```python
from build123d import *

# Parameters (mm, degrees)
CROQUIS1_R              = 1.75
SALIENTE_EXTRUIR1_DEPTH = 3
SALIENTE_EXTRUIR3_DEPTH = 10
CROQUIS4_W              = 70.682064062
CROQUIS4_H              = 54
CORTAR_EXTRUIR1_DEPTH   = 1.5


with BuildPart() as part:
    # Croquis1 → Saliente-Extruir1 (new body)
    with BuildSketch(Plane(origin=(0, 0, 0), x_dir=(1, 0, 0), z_dir=(0, 1, 0))):
        with BuildLine():
            Line((0, 35), (-75, 35))
            Line((-75, 35), (-75, -35))
            Line((-75, -35), (0, -35))
            ThreePointArc((0, -35), (35, 0), (0, 35))
        make_face()
        with Locations(Location((-72, 32, 0), (0, 0, 270))):
            Circle(CROQUIS1_R, mode=Mode.SUBTRACT)
        with Locations(Location((-72, -32, 0), (0, 0, 270))):
            Circle(CROQUIS1_R, mode=Mode.SUBTRACT)
        with Locations(Location((32, 0, 0), (0, 0, 270))):
            Circle(CROQUIS1_R, mode=Mode.SUBTRACT)
    extrude(amount=SALIENTE_EXTRUIR1_DEPTH)

    # Croquis3 → Saliente-Extruir3 (add)
    with BuildSketch(Plane(origin=(0, 3, 0), x_dir=(1, 0, 0), z_dir=(0, 1, 0))):
        Polygon((6.22052857, 28.5), (-63.77947143, 28.5), (-63.77947143, 25.5), (3.22052857, 25.5), (3.22052857, -25.5), (-63.77947143, -25.5), (-63.77947143, -28.5), (6.22052857, -28.5), align=None)
    extrude(amount=SALIENTE_EXTRUIR3_DEPTH)

    # Croquis4 → Cortar-Extruir1 (cut)
    with BuildSketch(Plane(origin=(0, 7, 0), x_dir=(1, 0, 0), z_dir=(0, 1, 0))):
        with Locations((-30.620503461, 0)):
            Rectangle(CROQUIS4_W, CROQUIS4_H)
    extrude(amount=CORTAR_EXTRUIR1_DEPTH, mode=Mode.SUBTRACT)


solid = part.part
```
The model under review builds one solid part; all positions refer to its coordinate system, in mm. A direction names the side the tool comes from. Round coordinates to 2 decimals unless told otherwise and drop trailing zeros. Order: outer loops, then holes, each group sorted by start corner. A loop starts at its lowest first (then second) coordinate and runs counter-clockwise, first axis right, second up.
Item 1: For pin 1 (3 mm diameter, centred on y = 5, z = 7.5, fed in from -X); pin 2 (1.3 mm diameter, centred on x = -40, y = 11.5, fed in from -Z); pin 3 (5 mm diameter, centred on x = -14, y = 9.5, fed in from +Z); pin 4 (5.5 mm diameter, centred on x = 32, z = 0, fed in from -Y), all flat-tipped, find the tip position at first contact; note any pin that passes through.
Working result:
pin 1: stops at x = 3.22
pin 2: stops at z = -28.5
pin 3: stops at z = 28.5
pin 4: stops at y = 0
Item 2: Add section D-D, the plane x = -23.5. State the section outline as (y, z) points, and give its area (4 significant figures).
Working result:
outline: (0, -35) - (3, -35) - (3, -28.5) - (13, -28.5) - (13, -25.5) - (8.5, -25.5) - (8.5, -27) - (7, -27) - (7, -25.5) - (3, -25.5) - (3, 25.5) - (7, 25.5) - (7, 27) - (8.5, 27) - (8.5, 25.5) - (13, 25.5) - (13, 28.5) - (3, 28.5) - (3, 35) - (0, 35) - close
area: 265.5 mm2
Item 3: To check wall thickness, follow probe 1 along Z at (x, y) = (-72, 2.45); probe 2 along Z at (x, y) = (-10, 10.75); probe 3 along X at (y, z) = (2, 0). State the ranges of each line that lie inside material, in increasing order.
Working result:
probe 1: z = -35 to -33.75, -30.25 to 30.25, 33.75 to 35
probe 2: z = -28.5 to -25.5, 25.5 to 28.5
probe 3: x = -75 to 30.25, 33.75 to 35
Item 4: Add section A-A, the plane x = -72. State the section outline as (y, z) points.
Working result:
outline: (0, -35) - (3, -35) - (3, -33.75) - (0, -33.75) - close; (0, -30.25) - (3, -30.25) - (3, 30.25) - (0, 30.25) - close; (0, 33.75) - (3, 33.75) - (3, 35) - (0, 35) - close
Item 5: Add section B-B, the plane z = -32. State the section outline as (x, y) points, and give its area (3 significant figures).
Working result:
outline: (-75, 0) - (-73.75, 0) - (-73.75, 3) - (-75, 3) - close; (-70.25, 0) - (14.18, 0) - (14.18, 3) - (-70.25, 3) - close
area: 257 mm2
Item 6: Draft analysis for pull direction Z (two halves, no side actions). For faces 1 (the flat face through (-21, 0, 0)), 2 (the cylindrical face through (34.99, 1.48, 0.77)), 3 (the flat face through (-30, 5, 25.5)), state which applies: released by +Z, released by -Z, zero draft, split by the parting line, or undercut.
Working result:
face 1: zero draft
face 2: split by the parting line
face 3: undercut
Item 7: Add section C-C, the plane y = 10.5. State the section outline as (x, z) points.
Working result:
outline: (-63.78, -28.5) - (6.22, -28.5) - (6.22, 28.5) - (-63.78, 28.5) - (-63.78, 25.5) - (3.22, 25.5) - (3.22, -25.5) - (-63.78, -25.5) - close
Item 8: Machinability: for faces 4 (the flat face through (6.221, 8, 0)), 5 (the flat face through (-29, 8, 28.5)), 6 (the flat face through (-63.779, 7.9, 27.3)), which of the approach directions +Z, -Z, +X, -X, +Y, -Y give a long, thin tool a straight path to every point of the face, cutting with its end or side? Answer none if there is none.
Working result:
face 4: +Z, -Z, +X, +Y
face 5: +Z, +X, -X, +Y
face 6: +Z, -Z, -X, +Y
